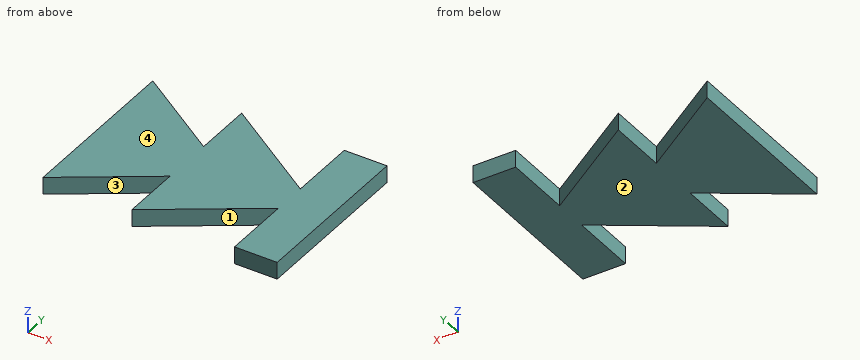
```python
from build123d import *

# Parameters (mm, degrees)
PAD003_DEPTH = 1
PAD004_DEPTH = 1
SKETCH010_W  = 2.5
SKETCH010_H  = 10
PAD005_DEPTH = 1


with BuildPart() as obj1:
    # Sketch012 → Pad003 (new body)
    with BuildSketch(Plane.XY):
        Polygon((-4.5, 5), (3, 0), (-4.5, -5), align=None)
    extrude(amount=PAD003_DEPTH)


with BuildPart() as obj1_1:
    # Body005 placement: moved
    add(obj1.part.moved(Location((-2.2, 0, 2))))


with BuildPart() as obj2:
    # Sketch011 → Pad004 (new body)
    with BuildSketch(Plane(origin=(1, 0, 0), x_dir=(1, 0, 0), z_dir=(0, 0, 1))):
        Polygon((-4.5, 5), (3, 0), (-4.5, -5), align=None)
    extrude(amount=PAD004_DEPTH)


with BuildPart() as obj2_1:
    # Body006 placement: moved
    add(obj2.part.moved(Location((2, 0, 2))))


with BuildPart() as obj3:
    # Sketch010 → Pad005 (new body)
    with BuildSketch(Plane.XY):
        with Locations((-4.45, 0)):
            Rectangle(SKETCH010_W, SKETCH010_H)
    extrude(amount=PAD005_DEPTH)


with BuildPart() as obj3_1:
    # Body007 placement: moved
    add(obj3.part.moved(Location((10.2, 0, 2))))

    # Fusion002: union obj1, obj2
    add(obj1_1.part)
    add(obj2_1.part)


solid = obj3_1.part
```
For this review, take the finished solid that the model builds, in its own axes (mm). Face numbers are marked on the shaded views. A direction names the side the tool comes from. Give positions to 0.01 mm unless a question says otherwise; leave off trailing zeros. Write each loop counter-clockwise with the first axis right and the second up, starting at its lowest first coordinate (ties: lowest second). Pieces come first, ordered by that corner, then holes. Notation, with made-up numbers: M -14.5,-37.75 L 39.5,-37.75 A16 cw 39.5,-17.75 Z; hole C -30.75,42 d5. An arc over 180 degrees is marked long. Answer as a JSON object with one key per item and string values. Group by question number.
Item 1: Consider section D-D on y = -1.25. Write out the cut boundary in (x, z) (3 decimals).
Item 2: Draft analysis for pull direction X (two halves, no side actions). For the marked faces 3 and 4, state which applies: +X half, -X half, draft (parallel to the pull), parting line (faces both ways), or undercut.
Item 3: For probe 1 along X at (y, z) = (4, 2.5); probe 2 along X at (y, z) = (-2.5, 2.45); probe 3 along Y at (x, z) = (0.25, 2.85), list the stretches that pass through material, from the lowest coordinate up. Write a range as [from, to].
Item 4: Consider section A-A on y = 2.25. Write out the cut boundary in (x, z) (3 decimals), plus the area to 4 significant figures.
Item 5: Consider section B-B on z = 2.55. Write out the cut boundary in (x, y), plus the area to 3 significant figures.
Item 6: Consider section C-C on x = 0. Write out the cut boundary in (y, z), plus the area to 3 significant figures.
Item 7: Tool access review of the marked faces 1 and 2: name each direction out of +Z, -Z, +X, -X, +Y, -Y from which nothing blocks a thin tool from reaching the whole face with its end or side.
Check result:
{
 "1": {"outline": "M -6.7,2 L 4.125,2 L 4.125,3 L -6.7,3 Z; M 4.5,2 L 7,2 L 7,3 L 4.5,3 Z"},
 "2": {"face 3": "undercut", "face 4": "draft"},
 "3": {"probe 1": "x = [-6.7, -5.2], [-1.5, 0], [4.5, 7]", "probe 2": "x = [-6.7, -2.95], [-1.5, 2.25], [4.5, 7]", "probe 3": "y = [-3.83, 3.83]"},
 "4": {"outline": "M -6.7,2 L -2.575,2 L -2.575,3 L -6.7,3 Z; M -1.5,2 L 2.625,2 L 2.625,3 L -1.5,3 Z; M 4.5,2 L 7,2 L 7,3 L 4.5,3 Z", "area": "10.75 mm^2"},
 "5": {"outline": "M -6.7,-5 L -1.5,-1.53 L -1.5,-5 L 4.5,-1 L 4.5,-5 L 7,-5 L 7,5 L 4.5,5 L 4.5,1 L -1.5,5 L -1.5,1.53 L -6.7,5 Z", "area": "95.0 mm^2"},
 "6": {"outline": "M -4,2 L 4,2 L 4,3 L -4,3 Z", "area": "8.00 mm^2"},
 "7": {"face 1": "+Z, -Z, -Y", "face 2": "-Z, +X, -X, +Y, -Y"}
}
